Input: part model. Units: mm. Frame: model coordinates. Round coordinates to 2 decimals unless told otherwise and drop trailing zeros. Loops run counter-clockwise (first coordinate to the right, second up) from the corner with the lowest first, then second, coordinate; pieces in that order, holes last. Notation, with made-up numbers: (11.5, 80.25) -> (34.5, 80.25) arc R18 ccw to (34.5, 113.25) -> close; hole circle Ø7 at (1, 47). An arc over 180 degrees is marked (long way). Answer as a JSON object with one key per item and string values.
```python
from build123d import *

# Parameters (mm, degrees)
BASE_FLANGE1_DEPTH      = 1200
SKETCH6_W               = 5
SKETCH6_H               = 17
CUT_EXTRUDE1_DEPTH      = 10
SKETCH7_W               = 5
SKETCH7_H               = 17.5
CUT_EXTRUDE2_DEPTH      = 1201.707645516
CUT_EXTRUDE3_DEPTH      = 1201.707645516
CUT_EXTRUDE3_DEPTH_BACK = 1201.707645516
SKETCH8_R               = 7.5


# Sheet-metal steps are written as plain solids
with BuildPart() as part:
    # Sketch1 → Base-Flange1 (new body)
    with BuildSketch(Plane(origin=(0, 0, 0), x_dir=(1, 0, 0), z_dir=(0, 1, 0))):
        with BuildLine():
            Line((36.7, 15), (36.7, 0.7))
            ThreePointArc((36.7, 0.7), (36.494974747, 0.205025253), (36, 0))
            Line((36, 0), (0.7, 0))
            ThreePointArc((0.7, 0), (0.205025253, 0.205025253), (0, 0.7))
            Line((0, 0.7), (0, 15))
            Line((0, 15), (-1.2, 15))
            Line((-1.2, 15), (-1.2, 0.7))
            ThreePointArc((-1.2, 0.7), (-0.643502884, -0.643502884), (0.7, -1.2))
            Line((0.7, -1.2), (36, -1.2))
            ThreePointArc((36, -1.2), (37.343502884, -0.643502884), (37.9, 0.7))
            Line((37.9, 0.7), (37.9, 15))
            Line((37.9, 15), (36.7, 15))
        make_face()
    extrude(amount=BASE_FLANGE1_DEPTH)

    # Sketch6 → Cut-Extrude1 (cut)
    with BuildSketch(Plane.ZY.offset(1.2)):
        with Locations((-12.5, 1191.5)):
            Rectangle(SKETCH6_W, SKETCH6_H)
        with Locations((-12.5, 8.5)):
            Rectangle(SKETCH6_W, SKETCH6_H)
    extrude(amount=-CUT_EXTRUDE1_DEPTH, mode=Mode.SUBTRACT)

    # Sketch7 → Cut-Extrude2 (cut, through all)
    with BuildSketch(Plane.XY.offset(1.2)):
        with Locations((1.3, 8.75)):
            Rectangle(SKETCH7_W, SKETCH7_H)
        with Locations((1.3, 1191.25)):
            Rectangle(SKETCH7_W, SKETCH7_H)
    extrude(amount=-CUT_EXTRUDE2_DEPTH, mode=Mode.SUBTRACT)

    # Sketch8 → Cut-Extrude3 (cut, two sides: drawn at the far end of the back side and taken through both)
    with BuildSketch(Plane.XY.offset(1.2).offset(-CUT_EXTRUDE3_DEPTH_BACK)):
        with Locations(Location((19.9, 126, 0), (0, 0, 180))):
            Circle(SKETCH8_R)
        with Locations(Location((19.9, 252, 0), (0, 0, 180))):
            Circle(SKETCH8_R)
        with Locations(Location((19.9, 378, 0), (0, 0, 180))):
            Circle(SKETCH8_R)
        with Locations(Location((19.9, 1074, 0), (0, 0, 180))):
            Circle(SKETCH8_R)
        with Locations(Location((19.9, 948, 0), (0, 0, 180))):
            Circle(SKETCH8_R)
        with Locations(Location((19.9, 822, 0), (0, 0, 180))):
            Circle(SKETCH8_R)
        with Locations(Location((19.9, 696, 0), (0, 0, 180))):
            Circle(SKETCH8_R)
        with Locations(Location((19.9, 537, 0), (0, 0, 180))):
            Circle(SKETCH8_R)
    extrude(amount=CUT_EXTRUDE3_DEPTH + CUT_EXTRUDE3_DEPTH_BACK, mode=Mode.SUBTRACT)


solid = part.part
```
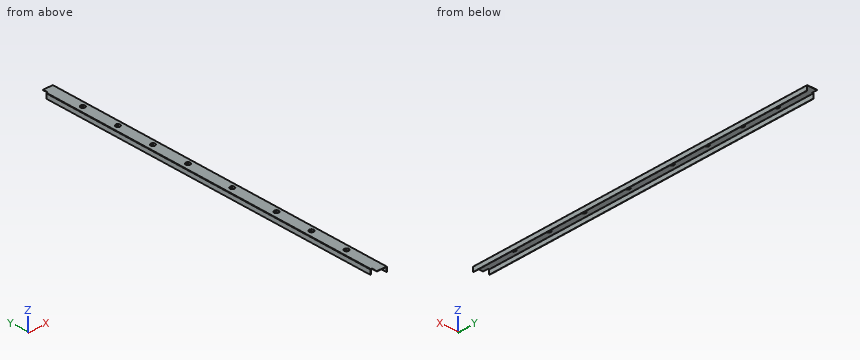
1) Contact query for flat-ended pins moving along their axis: P1, Ø4, axis at x = 1, z = -3.5, coming from the -Y side; P2, Ø17, axis at x = 19.9, y = 1074, coming from the -Z side; P3, Ø9, axis at x = 19.9, y = 537, coming from the -Z side; P4, Ø1.3, axis at y = 1192, z = 0.5, coming from the -X side. Output: stop coordinate, or through.
Output:
{"P1": "stops at y = 17.5", "P2": "stops at z = 0", "P3": "passes through", "P4": "stops at x = 3.8"}
2) Section B-B, the plane y = 228. Output: boundary loops of the cut face in (x, z), plus the area to 3 significant figures.
Output:
{"outline": "(-1.2, -15) -> (0, -15) -> (0, -0.7) arc R0.7 cw to (0.7, 0) -> (36, 0) arc R0.7 cw to (36.7, -0.7) -> (36.7, -15) -> (37.9, -15) -> (37.9, -0.7) arc R1.9 ccw to (36, 1.2) -> (0.7, 1.2) arc R1.9 ccw to (-1.2, -0.7) -> close", "area": "81.6 mm^2"}
3) Section A-A, the plane z = -12. Output: boundary loops of the cut face in (x, y).
Output:
{"outline": "(-1.2, 17.5) -> (0, 17.5) -> (0, 1182.5) -> (-1.2, 1182.5) -> close; (36.7, 0) -> (37.9, 0) -> (37.9, 1200) -> (36.7, 1200) -> close"}
4) Ray query, probe 1 along X at (y, z) = (916.5, -13.5); probe 2 along Z at (x, y) = (11, 366); probe 3 along X at (y, z) = (537, 0.4). Return the intervals inside material, ascending.
Output:
{"probe 1": "x = -1.2 to 0, 36.7 to 37.9", "probe 2": "z = 0 to 1.2", "probe 3": "x = -0.85 to 12.4, 27.4 to 37.55"}
